```python
from build123d import *

# Parameters (mm, degrees)
BOX006_W          = 1
BOX006_H          = 6
BOX006_DEPTH      = 4
BOX005_W          = 9
BOX005_H          = 1
BOX005_DEPTH      = 1
CYLINDER144_R     = 0.8
CYLINDER144_DEPTH = 10
CYLINDER136_R     = 0.2
CYLINDER136_DEPTH = 9
CYLINDER_R        = 1.1
CYLINDER_DEPTH    = 4
CYLINDER139_R     = 1.1
CYLINDER139_DEPTH = 4
CYLINDER138_R     = 0.165
CYLINDER138_DEPTH = 8
CYLINDER143_R     = 0.8
CYLINDER143_DEPTH = 10
BOX003_W          = 2.7
BOX003_H          = 4
BOX003_DEPTH      = 1.8
BOX004_W          = 2.7
BOX004_H          = 4
BOX004_DEPTH      = 1.8
CYLINDER142_R     = 2.5
CYLINDER142_DEPTH = 1.8
CYLINDER141_R     = 2.5
CYLINDER141_DEPTH = 1.8
CYLINDER140_R     = 0.35
CYLINDER140_DEPTH = 1
BOX_W             = 10
BOX_H             = 0.75
BOX_DEPTH         = 0.6
BOX002_W          = 11
BOX002_H          = 4
BOX002_DEPTH      = 1
BOX001_W          = 14
BOX001_H          = 6
BOX001_DEPTH      = 1


with BuildPart() as cube003:
    # Box006 → Box006 (new body)
    with BuildSketch(Plane(origin=(0, 3, -1), x_dir=(1, 0, 0), z_dir=(0, 0, 1))):
        with Locations((0.5, 3)):
            Rectangle(BOX006_W, BOX006_H)
    extrude(amount=BOX006_DEPTH)


with BuildPart() as cube002:
    # Box005 → Box005 (new body)
    with BuildSketch(Plane(origin=(-5, 4, -0.3), x_dir=(1, 0, 0), z_dir=(0, 0, 1))):
        with Locations((4.5, 0.5)):
            Rectangle(BOX005_W, BOX005_H)
    extrude(amount=BOX005_DEPTH)


with BuildPart() as cylinder001:
    # Cylinder144 → Cylinder144 (new body)
    with BuildSketch(Plane(origin=(6.3, -2.8, -1), x_dir=(1, 0, 0), z_dir=(0, 0, 1))):
        Circle(CYLINDER144_R)
    extrude(amount=CYLINDER144_DEPTH)


with BuildPart() as bowtienozzle:
    # Cylinder136 → Cylinder136 (new body)
    with BuildSketch(Plane.XY):
        Circle(CYLINDER136_R)
    extrude(amount=CYLINDER136_DEPTH)


with BuildPart() as mountinghole1:
    # Cylinder → Cylinder (new body)
    with BuildSketch(Plane(origin=(-5, 0, -1), x_dir=(1, 0, 0), z_dir=(0, 0, 1))):
        Circle(CYLINDER_R)
    extrude(amount=CYLINDER_DEPTH)


with BuildPart() as mountinghole2:
    # Cylinder139 → Cylinder139 (new body)
    with BuildSketch(Plane(origin=(5, 0, -1), x_dir=(1, 0, 0), z_dir=(0, 0, 1))):
        Circle(CYLINDER139_R)
    extrude(amount=CYLINDER139_DEPTH)


with BuildPart() as fusion001:
    # Cylinder138 → Cylinder138 (new body)
    with BuildSketch(Plane(origin=(0, 0, 0), x_dir=(1, 0, 0), z_dir=(0, 1, 0))):
        Circle(CYLINDER138_R)
    extrude(amount=CYLINDER138_DEPTH)

    # Fusion001: union BowTieNozzle, MountingHole1, MountingHole2
    add(bowtienozzle.part)
    add(mountinghole1.part)
    add(mountinghole2.part)


with BuildPart() as fusion003:
    # Cylinder143 → Cylinder143 (new body)
    with BuildSketch(Plane(origin=(-6.3, -2.8, -1), x_dir=(1, 0, 0), z_dir=(0, 0, 1))):
        Circle(CYLINDER143_R)
    extrude(amount=CYLINDER143_DEPTH)

    # Fusion003: union Cylinder001, Fusion001
    add(cylinder001.part)
    add(fusion001.part)


with BuildPart() as cube:
    # Box003 → Box003 (new body)
    with BuildSketch(Plane(origin=(4.8, -4, -0.3), x_dir=(1, 0, 0), z_dir=(0, 0, 1))):
        with Locations((1.35, 2)):
            Rectangle(BOX003_W, BOX003_H)
    extrude(amount=BOX003_DEPTH)


with BuildPart() as cube001:
    # Box004 → Box004 (new body)
    with BuildSketch(Plane(origin=(-7.5, -4, -0.3), x_dir=(1, 0, 0), z_dir=(0, 0, 1))):
        with Locations((1.35, 2)):
            Rectangle(BOX004_W, BOX004_H)
    extrude(amount=BOX004_DEPTH)


with BuildPart() as obj1:
    # Cylinder142 → Cylinder142 (new body)
    with BuildSketch(Plane(origin=(5, 0, -0.3), x_dir=(1, 0, 0), z_dir=(0, 0, 1))):
        Circle(CYLINDER142_R)
    extrude(amount=CYLINDER142_DEPTH)


with BuildPart() as obj2:
    # Cylinder141 → Cylinder141 (new body)
    with BuildSketch(Plane(origin=(-5, 0, -0.3), x_dir=(1, 0, 0), z_dir=(0, 0, 1))):
        Circle(CYLINDER141_R)
    extrude(amount=CYLINDER141_DEPTH)


with BuildPart() as nozzle_od:
    # Cylinder140 → Cylinder140 (new body)
    with BuildSketch(Plane.XY.offset(0.3)):
        Circle(CYLINDER140_R)
    extrude(amount=CYLINDER140_DEPTH)


with BuildPart() as fusion:
    # Box → Box (new body)
    with BuildSketch(Plane(origin=(-5, -0.375, -0.3), x_dir=(1, 0, 0), z_dir=(0, 0, 1))):
        with Locations((5, 0.375)):
            Rectangle(BOX_W, BOX_H)
    extrude(amount=BOX_DEPTH)

    # Fusion: union obj1, obj2, Nozzle_OD
    add(obj1.part)
    add(obj2.part)
    add(nozzle_od.part)


with BuildPart() as supportsubtract:
    # Box002 → Box002 (new body)
    with BuildSketch(Plane(origin=(-5.5, 0, -0.3), x_dir=(1, 0, 0), z_dir=(0, 0, 1))):
        with Locations((5.5, 2)):
            Rectangle(BOX002_W, BOX002_H)
    extrude(amount=BOX002_DEPTH)


with BuildPart() as cut002:
    # Box001 → Box001 (new body)
    with BuildSketch(Plane(origin=(-7, 0, -0.3), x_dir=(1, 0, 0), z_dir=(0, 0, 1))):
        with Locations((7, 3)):
            Rectangle(BOX001_W, BOX001_H)
    extrude(amount=BOX001_DEPTH)

    # Cut: cut SupportSubtract
    add(supportsubtract.part, mode=Mode.SUBTRACT)

    # Fusion002: union Cube, Cube001, Fusion
    add(cube.part)
    add(cube001.part)
    add(fusion.part)

    # Cut001: cut Fusion003
    add(fusion003.part, mode=Mode.SUBTRACT)

    # Fusion004: union Cube002
    add(cube002.part)

    # Cut002: cut Cube003
    add(cube003.part, mode=Mode.SUBTRACT)


solid = cut002.part
```
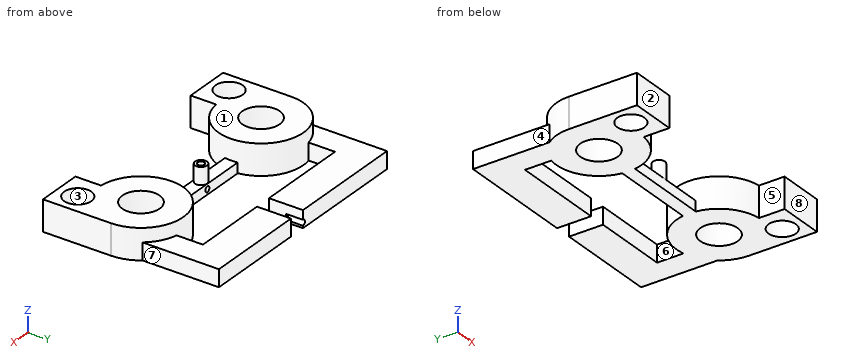
Read the model definition and answer for the solid it produces. Units are mm, in the model's axes. Face numbers are marked on the shaded views. A direction names the side the tool comes from. Coordinates: 2 decimals unless noted, no trailing zeros. Loops run counter-clockwise (first coordinate to the right, second up) from the corner with the lowest first, then second, coordinate; pieces in that order, holes last.
(1) The part is cut by section B-B (x = -3). Determine the outline of the cut face in (y, z), and give its area (3 significant figures).
Solution:
outline: (-1.5, -0.3) - (1.5, -0.3) - (1.5, 1.5) - (-1.5, 1.5) - close; (4, -0.3) - (6, -0.3) - (6, 0.7) - (4, 0.7) - close
area: 7.40 mm2
(2) A tool of negligible diameter and unlimited length cuts with its end or side. For the marked faces 4, 5, 6, 7 and 8, from which of +Z, -Z, +X, -X, +Y, -Y can it reach the whole face along a straight path? Write none if from no direction.
Solution:
face 4: +Z, -Z, -X, +Y
face 5: +Z, -Z, -Y
face 6: +Z, -Z
face 7: +Z, -Z, +X, +Y
face 8: +Z, -Z, +X, -X, -Y
(3) The part is cut by section D-D (y = -1.5). Determine the outline of the cut face in (x, z), and give its area (3 significant figures).
Solution:
outline: (-7.5, -0.3) - (-3, -0.3) - (-3, 1.5) - (-7.5, 1.5) - close; (3, -0.3) - (7.5, -0.3) - (7.5, 1.5) - (3, 1.5) - close
area: 16.2 mm2
(4) Consider line 1 along X through (y, z) = (4.75, 0.15); line 2 along X through (y, z) = (0.2, 0) (3 decimals); line 3 along X through (y, z) = (-3.25, 0.55). Determine where each line is inside the solid, lowest interval first.
Solution:
line 1: x = -7 to 0, 1 to 7
line 2: x = -7.492 to -6.082, -3.918 to -0.165, 0.165 to 3.918, 6.082 to 7.492
line 3: x = -7.5 to -6.96, -5.64 to -4.8, 4.8 to 5.64, 6.96 to 7.5
(5) The mould has two halves that part along Y. Classify the marked faces 1, 2 and 3: released by +Y, released by -Y, zero draft, split by the parting line, or undercut.
Solution:
face 1: zero draft
face 2: released by -Y
face 3: undercut
(6) The part is cut by section A-A (z = 0.95). Determine the outline of the cut face in (x, y).
Solution:
outline: (-7.5, -4) - (-4.8, -4) - (-4.8, -2.49) arc R2.5 ccw (long way) to (-7.5, 0) - close; circle Ø0.7 at (0, 0); (4.8, -4) - (7.5, -4) - (7.5, 0) arc R2.5 ccw (long way) to (4.8, -2.49) - close; hole circle Ø1.6 at (-6.3, -2.8); hole circle Ø2.2 at (-5, 0); hole circle Ø0.4 at (0, 0); hole circle Ø2.2 at (5, 0); hole circle Ø1.6 at (6.3, -2.8)
(7) The part is cut by section C-C (x = -5). Determine the outline of the cut face in (y, z).
Solution:
outline: (-4, -0.3) - (-1.1, -0.3) - (-1.1, 1.5) - (-4, 1.5) - close; (1.1, -0.3) - (2.5, -0.3) - (2.5, 1.5) - (1.1, 1.5) - close; (4, -0.3) - (6, -0.3) - (6, 0.7) - (4, 0.7) - close
(8) Flat-ended cylindrical pins translate along their axes: pin 1 Ø0.5 at (y, z) = (3, 0.5) entering from -X; pin 2 Ø0.5 at (x, z) = (1, 0) entering from -Y (3 decimals); pin 3 Ø0.8 at (x, z) = (2.5, 0) entering from -Y. Find the tip coordinate at first contact, or state that the pin passes through.
Solution:
pin 1: stops at x = -7
pin 2: stops at y = -0.375
pin 3: stops at y = -1.36
